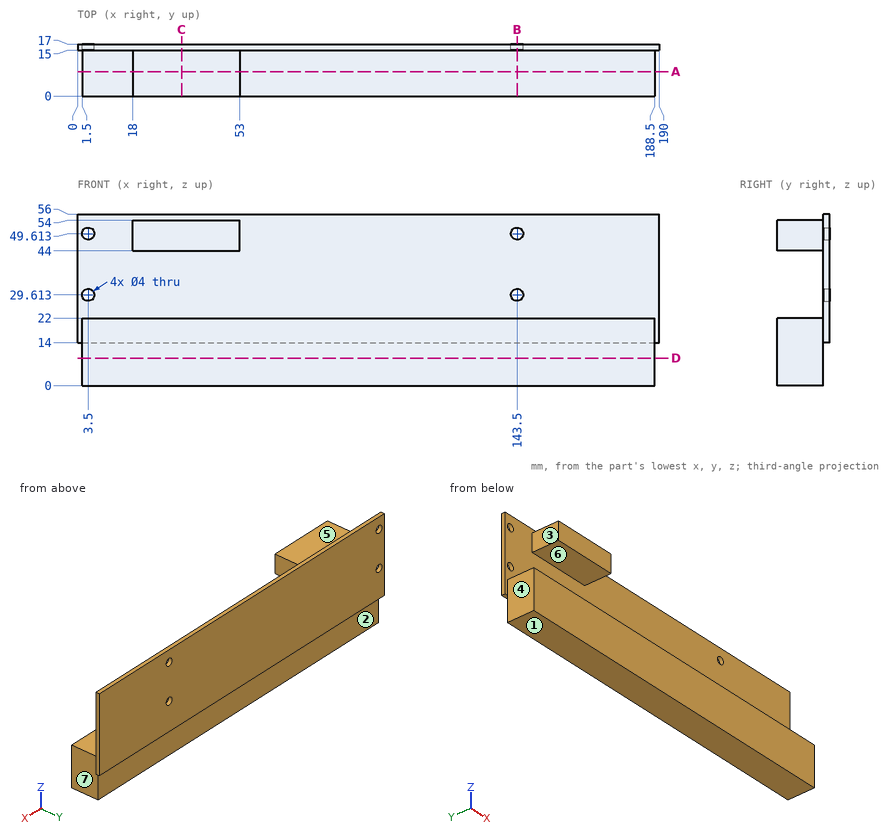
Could you check a few things on this drawing? It's one solid part, dimensions in mm from its lowest x, y, z. A direction names the side the tool comes from. Give positions to 0.01 mm unless a question says otherwise; leave off trailing zeros. Order: outer loops, then holes, each group sorted by start corner. A loop starts at its lowest first (then second) coordinate and runs counter-clockwise, first axis right, second up. Notation, with made-up numbers: (29.25, 40) - (73.25, 40) arc R18 cw to (73.25, 64) - close; hole circle Ø11 at (-5.5, -14). An arc over 180 degrees is marked (long way). Return JSON: item names as keys, results as strings. Group by question number.
Q1. Suppose I cut it at D-D, the plane z = 9. Please give me the cut outline in (x, y), and give its area (4 significant figures).
Q2. Thinking about a two-plate mould opening in Z: for the marked faces 5, 6 and 7, which applies, pulls with the +Z half, pulls with the -Z half, needs draft (parallel to the pull), parting line crosses it, or undercut?
Q3. Please list where these lines run through material, in increasing order: line 1 along Z through (x, y) = (3.5, 16.3); line 2 along Z through (x, y) = (44.5, 14.75); line 3 along Y through (x, z) = (12.5, 5). Write a range as [from, to].
Q4. Suppose I cut it at A-A, the plane y = 8. Please give me the cut outline in (x, z), and give its area (3 significant figures).
Q5. Suppose I cut it at B-B, the plane x = 143.5. Please give me the cut outline in (y, z), and give its area (3 significant figures).
Q6. Will these pins go through, and if not, where does the flat tip stop? pin 1 Ø4.5 at (x, z) = (3.5, 29.61) entering from -Y; pin 2 Ø3 at (y, z) = (11, 47.5) entering from +X; pin 3 Ø1 at (x, y) = (22, 4.5) entering from +Z.
Q7. Suppose I cut it at C-C, the plane x = 34. Please give me the cut outline in (y, z), and give its area (3 significant figures).
Q8. Which directions (+Z, -Z, +X, -X, +Y, -Y) give clear straight access to the entire face, cutting with the end or side of a thin tool? Please do the marked faces 1, 2, 3 and 4.
Resolved:
{
 "1": {"outline": "(1.5, 0) - (188.5, 0) - (188.5, 15) - (1.5, 15) - close", "area": "2,805 mm2"},
 "2": {"face 5": "pulls with the +Z half", "face 6": "undercut", "face 7": "needs draft"},
 "3": {"line 1": "z = [14, 27.61], [31.61, 47.61], [51.61, 56]", "line 2": "z = [0, 22], [44, 54]", "line 3": "y = [0, 15]"},
 "4": {"outline": "(1.5, 0) - (188.5, 0) - (188.5, 22) - (1.5, 22) - close; (18, 44) - (53, 44) - (53, 54) - (18, 54) - close", "area": "4,460 mm2"},
 "5": {"outline": "(0, 0) - (15, 0) - (15, 14) - (17, 14) - (17, 27.61) - (15, 27.61) - (15, 22) - (0, 22) - close; (15, 31.61) - (17, 31.61) - (17, 47.61) - (15, 47.61) - close; (15, 51.61) - (17, 51.61) - (17, 56) - (15, 56) - close", "area": "398 mm2"},
 "6": {"pin 1": "stops at y = 15", "pin 2": "stops at x = 53", "pin 3": "stops at z = 54"},
 "7": {"outline": "(0, 0) - (15, 0) - (15, 14) - (17, 14) - (17, 56) - (15, 56) - (15, 54) - (0, 54) - (0, 44) - (15, 44) - (15, 22) - (0, 22) - close", "area": "564 mm2"},
 "8": {"face 1": "-Z, +X, -X, +Y, -Y", "face 2": "-Z, +X, -X, +Y", "face 3": "+Z, -X, -Y", "face 4": "+Z, -Z, -X, -Y"}
}
